CAD build for the part. Positions are in the model's coordinates, mm. Give positions to 0.01 mm unless a question says otherwise; leave off trailing zeros. Order: outer loops, then holes, each group sorted by start corner. A loop starts at its lowest first (then second) coordinate and runs counter-clockwise, first axis right, second up. Notation, with made-up numbers: (-40, 23) -> (11, 23) arc R16 cw to (11, 46) -> close; hole circle Ø7 at (-19.5, 10.25). An arc over 180 degrees is marked (long way). Answer as CSV lines item,"result".
Autodesk Inventor part; units mm, degrees
ref_plane "YZ Plane" through (0, 0, 0) normal (1, 0, 0) x (0, 1, 0)
ref_plane "XZ Plane" through (0, 0, 0) normal (0, 1, 0) x (-1, 0, 0)
ref_plane "XY Plane" through (0, 0, 0) normal (0, 0, 1) x (1, 0, 0)
sketch "Boceto1" plane through (0, 0, 0) normal (0, 0, 1) x (1, 0, 0)
  line L0 (3.3269, 0.8317) -> (3.3269, 50.8317)
  line L1 (3.3269, 50.8317) -> (153.3269, 50.8317)
  line L2 (153.3269, 50.8317) -> (153.3269, 0.8317)
  line L3 (153.3269, 0.8317) -> (3.3269, 0.8317)
  point P0 (0, 0)
  dimension "d0" = 150
  dimension "d1" = 50
extrude "Extrusión1" add sketch "Boceto1" along normal mid plane 20
sketch "Boceto3" plane through (0, 0, 10) normal (0, 0, 1) x (1, 0, 0)
  circle A0 centre (146.5928, 38.3317) radius 3.5
  circle A1 centre (146.5928, 13.3317) radius 3.5
  line L0 (3.3269, 50.8317) -> (153.3269, 50.8317)
  circle A2 centre (146.5928, 38.3317) radius 4.5
  circle A3 centre (146.5928, 13.3317) radius 4.5
  line L1 (153.3269, 50.8317) -> (3.3269, 50.8317)
  circle A4 centre (10.0609, 38.3317) radius 3.5
  circle A5 centre (10.0609, 13.3317) radius 3.5
  circle A6 centre (10.0609, 38.3317) radius 4.5
  circle A7 centre (10.0609, 13.3317) radius 4.5
  point P0 (0, 0)
  dimension "d8" = 7
  dimension "d9" = 7
  dimension "d10" = 25
  dimension "d11" = 12.5
  dimension "d12" = 9
  dimension "d13" = 9
hole "Agujero1" at (10.0609, 38.3317, 10) at (10.0609, 13.3317, 10) at (146.5928, 38.3317, 10) at (146.5928, 13.3317, 10) direction (0, 0, -1) diameter 7 depth 40 countersink diameter 9 countersink angle 82
properties part number "soporte_rueca"
1) Band-saw the part on B-B, the plane y = 11.5. Give the number of separate pieces and of enclosed holes in the cut face, then the cut area to 3 significant figures.
Data:
separate pieces,"3"
enclosed holes,"0"
area,"2,760 mm2"
2) Pin check, flat tip, straight feed: P1, Ø5.5, axis at x = 146.59, y = 38.33, coming from the +Z side. Stop position of the tip, or through.
Data:
P1,"passes through"
3) Wall check: line 1 along X through (y, z) = (16, 6); line 2 along X through (y, z) = (14.5, 4.5). Give the ranges that are in metal, low to high. Write a range as [from, to].
Data:
line 1,"x = [3.33, 7.8], [12.33, 144.33], [148.86, 153.33]"
line 2,"x = [3.33, 6.76], [13.36, 143.29], [149.89, 153.33]"
4) Pull direction Y, two halves, no side cores. Call faces 1 (the cylindrical face through (150.01, 14.09, -0.71)), 2 (the cylindrical face through (6.59, 13.79, -0.71)), 3 (the flat face through (153.327, 26, 0)), 4 (the flat face through (79, 0.832, 0)): pulls with the +Y half, pulls with the -Y half, needs draft (parallel to the pull), parting line crosses it, or undercut.
Data:
face 1,"undercut"
face 2,"undercut"
face 3,"needs draft"
face 4,"pulls with the -Y half"
5) Band-saw the part on A-A, the plane z = -2.25. Write the cut outline in (x, y), then the cut area to 3 significant figures.
Data:
outline,"(3.33, 0.83) -> (153.33, 0.83) -> (153.33, 50.83) -> (3.33, 50.83) -> close; hole circle Ø7 at (10.06, 13.33); hole circle Ø7 at (10.06, 38.33); hole circle Ø7 at (146.59, 13.33); hole circle Ø7 at (146.59, 38.33)"
area,"7,350 mm2"
